Work out the finished part from the listing and answer in its coordinate system (mm). Face numbers are marked on the shaded views. A direction names the side the tool comes from. Round coordinates to 2 decimals unless told otherwise and drop trailing zeros. Write each loop counter-clockwise with the first axis right and the second up, starting at its lowest first coordinate (ties: lowest second). Pieces come first, ordered by that corner, then holes. Notation, with made-up numbers: (41, -8.5) -> (49, -8.5) arc R11 cw to (49, 4.5) -> close; hole circle Ø5 at (89.5, 3.25). An arc over 180 degrees is marked (long way). Answer as a JSON object with one key per item and string values. Group by question number.
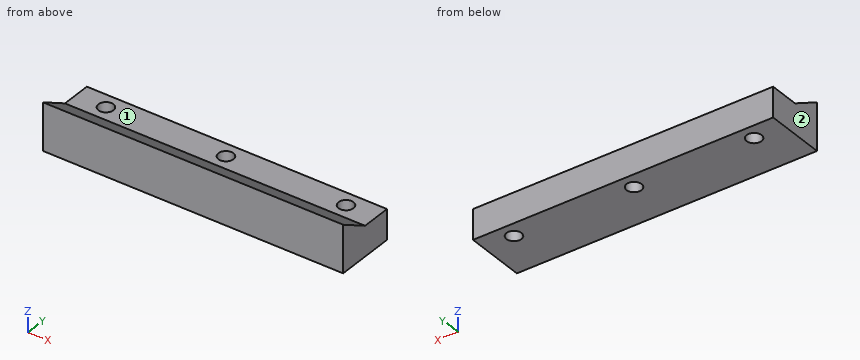
from build123d import *

# Parameters (mm, degrees)
F1_DEPTH = 127
F3_DEPTH = 12.701


with BuildPart() as f1:
    # F0 (on Right) → F1 (new body)
    with BuildSketch(Plane.YZ):
        Polygon((0, 20.032348), (0, 0), (25.4, 0), (25.4, 12.7), (12.7, 12.7), align=None)
    extrude(amount=-F1_DEPTH)

    # F2 (on face) → F3 (cut, through all)
    with BuildSketch(Plane.XY.offset(12.7)):
        with BuildLine():
            ThreePointArc((-111.125, 19.05), (-114.3, 22.225), (-117.475, 19.05))
            Line((-117.475, 19.05), (-111.125, 19.05))
        make_face()
        with BuildLine():
            ThreePointArc((-9.525, 19.05), (-12.7, 22.225), (-15.875, 19.05))
            Line((-15.875, 19.05), (-9.525, 19.05))
        make_face()
        with BuildLine():
            Line((-9.525, 19.05), (-15.875, 19.05))
            ThreePointArc((-15.875, 19.05), (-12.7, 15.875), (-9.525, 19.05))
        make_face()
        with BuildLine():
            ThreePointArc((-60.325, 19.05), (-63.5, 22.225), (-66.675, 19.05))
            Line((-66.675, 19.05), (-60.325, 19.05))
        make_face()
        with BuildLine():
            Line((-60.325, 19.05), (-66.675, 19.05))
            ThreePointArc((-66.675, 19.05), (-63.5, 15.875), (-60.325, 19.05))
        make_face()
        with BuildLine():
            Line((-111.125, 19.05), (-117.475, 19.05))
            ThreePointArc((-117.475, 19.05), (-114.3, 15.875), (-111.125, 19.05))
        make_face()
    extrude(amount=-F3_DEPTH, mode=Mode.SUBTRACT)


solid = f1.part
1) A cutting plane is placed at D-D on x = -12.7. Determine the outline of the cut face in (y, z) (3 decimals).
2) A cutting plane is placed at A-A on y = 19.05. Determine the outline of the cut face in (x, z) (3 decimals).
3) A cutting plane is placed at B-B on z = 7.75. Determine the outline of the cut face in (x, y) (3 decimals).
4) A cutting plane is placed at C-C on x = -65. Determine the outline of the cut face in (y, z).
5) Straight lines are drawn through the part: L1, parallel to X at y = 19.05, z = 6.75 (3 decimals); L2, parallel to Y at x = -63.5, z = 5 (3 decimals); L3, parallel to Z at x = -33.5, y = 15.5. For each, find the intervals that lie inside material, in ascending order.
6) A tool of negligible diameter and unlimited length cuts with its end or side. For the marked faces 1 and 2, from which of +Z, -Z, +X, -X, +Y, -Y can it reach the whole face along a straight path? Write none if from no direction.
7) Each of these flat-tipped pins is pushed along its axis until it touches: P1, Ø6.5, axis at x = -32.5, y = 18.5, coming from the +Z side; P2, Ø4, axis at x = -12.7, y = 19.05, coming from the +Z side; P3, Ø4, axis at x = -98.5, y = 5.5, coming from the +Z side. Where does it stop, or does it pass through?
Established:
{
 "1": {"outline": "(0, 0) -> (15.875, 0) -> (15.875, 12.7) -> (12.7, 12.7) -> (0, 20.032) -> close; (22.225, 0) -> (25.4, 0) -> (25.4, 12.7) -> (22.225, 12.7) -> close"},
 "2": {"outline": "(-127, 0) -> (-117.475, 0) -> (-117.475, 12.7) -> (-127, 12.7) -> close; (-111.125, 0) -> (-66.675, 0) -> (-66.675, 12.7) -> (-111.125, 12.7) -> close; (-60.325, 0) -> (-15.875, 0) -> (-15.875, 12.7) -> (-60.325, 12.7) -> close; (-9.525, 0) -> (0, 0) -> (0, 12.7) -> (-9.525, 12.7) -> close"},
 "3": {"outline": "(-127, 0) -> (0, 0) -> (0, 25.4) -> (-127, 25.4) -> close; hole circle Ø6.35 at (-114.3, 19.05); hole circle Ø6.35 at (-63.5, 19.05); hole circle Ø6.35 at (-12.7, 19.05)"},
 "4": {"outline": "(0, 0) -> (16.25, 0) -> (16.25, 12.7) -> (12.7, 12.7) -> (0, 20.03) -> close; (21.85, 0) -> (25.4, 0) -> (25.4, 12.7) -> (21.85, 12.7) -> close"},
 "5": {"L1": "x = -127 to -117.475, -111.125 to -66.675, -60.325 to -15.875, -9.525 to 0", "L2": "y = 0 to 15.875, 22.225 to 25.4", "L3": "z = 0 to 12.7"},
 "6": {"face 1": "+Z, +X, -X, +Y", "face 2": "+Z, -Z, -X, +Y, -Y"},
 "7": {"P1": "stops at z = 12.7", "P2": "passes through", "P3": "stops at z = 18.01"}
}
